```python
from build123d import *

# Parameters (mm, degrees)
SKETCH138_R     = 5
PAD002_DEPTH    = 2
SKETCH139_W     = 64
SKETCH139_H     = 1
SKETCH139_W_2   = 1.03067
SKETCH139_H_2   = 2.2409
SKETCH139_W_3   = 1.02889
SKETCH139_H_3   = 2.288
PAD003_DEPTH    = 65.5
SKETCH140_R     = 5
PAD004_DEPTH    = 2
SKETCH141_W     = 64
SKETCH141_H     = 1
PAD005_DEPTH    = 30
SKETCH144_W     = 28
SKETCH144_H     = 2
PAD007_DEPTH    = 15
SKETCH146_W     = 18.3
SKETCH146_H     = 4.3
POCKET028_DEPTH = 2
FILLET005_R     = 4
FILLET006_R     = 6
SKETCH147_R     = 0.65
POCKET029_DEPTH = 2
SKETCH149_W     = 3.03
SKETCH149_H     = 2.00511
SKETCH149_W_2   = 6
SKETCH149_H_2   = 3
SKETCH149_W_3   = 3.03002
SKETCH149_H_3   = 2.04501
PAD008_DEPTH    = 13.5
SKETCH150_W     = 90
SKETCH150_H     = 24
PAD009_DEPTH    = 2
FILLET007_R     = 9
FILLET008_R     = 5
SKETCH161_W     = 26
SKETCH161_H     = 18
PAD014_DEPTH    = 9
SKETCH162_W     = 23
SKETCH162_H     = 14.90769
SKETCH162_W_2   = 22.99998
SKETCH162_H_2   = 14.95065
POCKET035_DEPTH = 9.5
FILLET014_R     = 2
FILLET015_R     = 2
FILLET016_R     = 1
SKETCH163_R     = 0.75
POCKET036_DEPTH = 2


with BuildPart() as part:
    # Sketch138 → Pad002 (new body)
    with BuildSketch(Plane.XZ):
        with BuildLine():
            ThreePointArc((413.000007, 21.499985), (403.500007, 11.999985), (413.000007, 2.499985))
            Line((477.000007, 2.499985), (413.000007, 2.499985))
            ThreePointArc((477.000007, 2.499985), (486.500006, 11.999985), (477.000007, 21.499985))
            Line((413.000007, 21.499985), (477.000007, 21.499985))
        make_face()
        with Locations((414.971964, 12)):
            Circle(SKETCH138_R, mode=Mode.SUBTRACT)
        with Locations((434.971964, 12)):
            Circle(SKETCH138_R, mode=Mode.SUBTRACT)
        with Locations((454.971964, 12)):
            Circle(SKETCH138_R, mode=Mode.SUBTRACT)
        with Locations((474.982974, 12)):
            Circle(SKETCH138_R, mode=Mode.SUBTRACT)
    extrude(amount=PAD002_DEPTH)

    # Sketch139 (on Face10 of Pad002) → Pad003 (join)
    with BuildSketch(Plane.XZ.offset(2)):
        with Locations((445.000007, 3)):
            Rectangle(SKETCH139_W, SKETCH139_H)
        with Locations((404.084671, 12.02045)):
            Rectangle(SKETCH139_W_2, SKETCH139_H_2)
        with Locations((485.914449, 11.999413)):
            Rectangle(SKETCH139_W_3, SKETCH139_H_3)
    extrude(amount=PAD003_DEPTH)

    # Sketch140 (on Face24 of Pad003) → Pad004 (join)
    with BuildSketch(Plane.XZ.offset(67.5)):
        with BuildLine():
            ThreePointArc((413.000007, 21.499985), (403.500007, 11.999985), (413.000007, 2.499985))
            Line((477.000007, 2.499985), (413.000007, 2.499985))
            ThreePointArc((477.000007, 2.499985), (486.500006, 11.999985), (477.000007, 21.499985))
            Line((413.000007, 21.499985), (477.000007, 21.499985))
        make_face()
        with Locations((414.971964, 12)):
            Circle(SKETCH140_R, mode=Mode.SUBTRACT)
        with Locations((434.971964, 12)):
            Circle(SKETCH140_R, mode=Mode.SUBTRACT)
        with Locations((454.971964, 12)):
            Circle(SKETCH140_R, mode=Mode.SUBTRACT)
        with Locations((474.982974, 12)):
            Circle(SKETCH140_R, mode=Mode.SUBTRACT)
    extrude(amount=PAD004_DEPTH)

    # Sketch141 (on Face32 of Pad004) → Pad005 (join)
    with BuildSketch(Plane(origin=(0, 0, 0), x_dir=(1, 0, 0), z_dir=(0, 1, 0))):
        with Locations((445, -3.005366)):
            Rectangle(SKETCH141_W, SKETCH141_H)
    extrude(amount=PAD005_DEPTH)

    # Sketch144 (on Face35 of Pad005) → Pad007 (join)
    with BuildSketch(Plane(origin=(0, 0, 3.505366), x_dir=(-1, 0, 0), z_dir=(0, 0, 1))):
        with Locations((-445, -28)):
            Rectangle(SKETCH144_W, SKETCH144_H)
    extrude(amount=PAD007_DEPTH)

    # Sketch146 (on Face41 of Pad007) → Pocket028 (cut)
    with BuildSketch(Plane(origin=(0, 29, 0), x_dir=(1, 0, 0), z_dir=(0, 1, 0))):
        with Locations((444.99999, -12)):
            Rectangle(SKETCH146_W, SKETCH146_H)
    extrude(amount=-POCKET028_DEPTH, mode=Mode.SUBTRACT)

    # Fillet005
    fillet005_edges = [part.edges().sort_by_distance(p)[0] for p in [
        (431, 28, 18.505366),
        (459, 28, 18.505366),
    ]]
    fillet(fillet005_edges, radius=FILLET005_R)

    # Fillet006
    fillet006_edges = [part.edges().sort_by_distance(p)[0] for p in [
        (431, 28, 3.505366),
        (459, 28, 3.505366),
    ]]
    fillet(fillet006_edges, radius=FILLET006_R)

    # Sketch147 (on Face5 of Fillet006) → Pocket029 (cut)
    with BuildSketch(Plane(origin=(0, 29, 0), x_dir=(1, 0, 0), z_dir=(0, 1, 0))):
        with Locations((434.559988, -12)):
            Circle(SKETCH147_R)
        with Locations((455.43999, -12)):
            Circle(SKETCH147_R)
    extrude(amount=-POCKET029_DEPTH, mode=Mode.SUBTRACT)

    # Sketch149 (on Face52 of Pocket029) → Pad008 (join)
    with BuildSketch(Plane.XZ.offset(69.5)):
        with Locations((484.914989, 12.142557)):
            Rectangle(SKETCH149_W, SKETCH149_H)
        with Locations((445, 4.5)):
            Rectangle(SKETCH149_W_2, SKETCH149_H_2)
        with Locations((405.084996, 12.122505)):
            Rectangle(SKETCH149_W_3, SKETCH149_H_3)
        with Locations((445.000007, 19.5)):
            Rectangle(SKETCH149_W_2, SKETCH149_H_2)
    extrude(amount=PAD008_DEPTH)

    # Sketch150 (on Face70 of Pad008) → Pad009 (join)
    with BuildSketch(Plane.XZ.offset(83)):
        with Locations((444.999989, 12.25)):
            Rectangle(SKETCH150_W, SKETCH150_H)
    extrude(amount=PAD009_DEPTH)

    # Fillet007
    fillet007_edges = [part.edges().sort_by_distance(p)[0] for p in [
        (489.999989, -84, 24.25),
        (399.999989, -84, 24.25),
    ]]
    fillet(fillet007_edges, radius=FILLET007_R)

    # Fillet008
    fillet008_edges = [part.edges().sort_by_distance(p)[0] for p in [
        (489.999989, -84, 0.25),
        (399.999989, -84, 0.25),
    ]]
    fillet(fillet008_edges, radius=FILLET008_R)

    # Sketch161 (on Face1 of Fillet008) → Pad014 (join)
    with BuildSketch(Plane(origin=(0, -83, 0), x_dir=(1, 0, 0), z_dir=(0, 1, 0))):
        with Locations((467, -12.257592)):
            Rectangle(SKETCH161_W, SKETCH161_H)
        with Locations((422.99999, -12.250199)):
            Rectangle(SKETCH161_W, SKETCH161_H)
    extrude(amount=PAD014_DEPTH)

    # Sketch162 (on Face34 of Pad014) → Pocket035 (cut)
    with BuildSketch(Plane.XZ.offset(85)):
        with Locations((423.000006, 12.246182)):
            Rectangle(SKETCH162_W, SKETCH162_H)
        with Locations((466.999997, 12.225325)):
            Rectangle(SKETCH162_W_2, SKETCH162_H_2)
    extrude(amount=-POCKET035_DEPTH, mode=Mode.SUBTRACT)

    # Fillet014
    fillet014_edges = [part.edges().sort_by_distance(p)[0] for p in [
        (434.500006, -75.5, 12.246182),
        (455.500007, -75.5, 12.225325),
    ]]
    fillet(fillet014_edges, radius=FILLET014_R)

    # Fillet015
    fillet015_edges = [part.edges().sort_by_distance(p)[0] for p in [
        (455.500007, -81.25, 4.75),
        (434.500006, -81.25, 4.792337),
        (434.500006, -81.25, 19.700027),
        (455.500007, -81.25, 19.70065),
    ]]
    fillet(fillet015_edges, radius=FILLET015_R)

    # Fillet016
    fillet016_edges = [part.edges().sort_by_distance(p)[0] for p in [
        (411.500006, -81.25, 4.792337),
        (411.500006, -75.5, 12.246182),
        (411.500006, -81.25, 19.700027),
        (411.500006, -76.085786, 19.114241),
        (411.500006, -76.085786, 5.378123),
        (478.499987, -81.25, 4.75),
        (478.499987, -76.085786, 5.335786),
        (478.499987, -75.5, 12.225325),
        (478.499987, -76.085786, 19.114864),
        (478.499987, -81.25, 19.70065),
    ]]
    fillet(fillet016_edges, radius=FILLET016_R)

    # Sketch163 (on Face2 of Fillet016) → Pocket036 (cut)
    with BuildSketch(Plane.XZ.offset(85)):
        with Locations((403.000006, 19.8)):
            Circle(SKETCH163_R)
        with Locations((487.03999, 19.8)):
            Circle(SKETCH163_R)
        with Locations((402.069775, 3.2)):
            Circle(SKETCH163_R)
        with Locations((488.100007, 3.2)):
            Circle(SKETCH163_R)
    extrude(amount=-POCKET036_DEPTH, mode=Mode.SUBTRACT)


with BuildPart() as part_1:
    # Body015 placement: moved
    add(part.part.moved(Location((0, 182, 0))))


solid = part_1.part
```
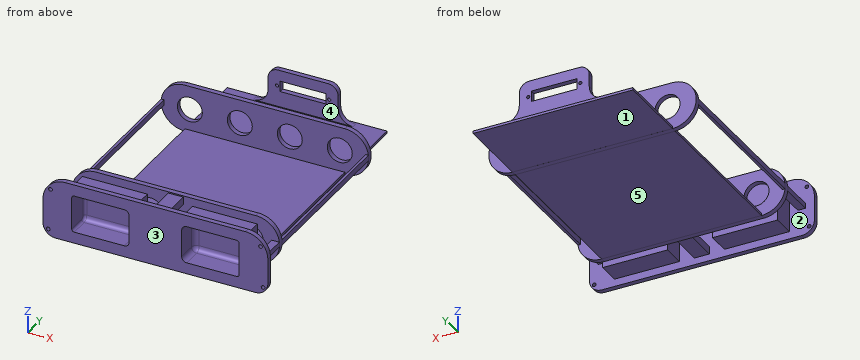
Check sheet for the modelled part. Datum: model origin and axes. Units: mm. Face numbers are marked on the shaded views. A direction names the side the tool comes from. Coordinates: 2 decimals unless noted, no trailing zeros. Loops run counter-clockwise (first coordinate to the right, second up) from the corner with the lowest first, then second, coordinate; pieces in that order, holes last.
1) Material ranges on probe 1 along X at (y, z) = (210.6, 12); probe 2 along Y at (x, z) = (405, 12.5); probe 3 along Y at (x, z) = (409, 10.5), recorded low to high.
2) Gauge pin test, flat ends, axial feed: pin 1 (5 mm diameter, centred on y = 131, z = 10, fed in from +X); pin 2 (1.5 mm diameter, centred on y = 111.5, z = 7.5, fed in from +X); pin 3 (7 mm diameter, centred on y = 103, z = 11.5, fed in from -X); pin 4 (13 mm diameter, centred on x = 474.98, z = 12, fed in from +Y). Record the tip position at first contact, or that the pin passes through.
3) Release check for a two-part mould opening along X. For the marked faces 1 and 2 record: released by +X, released by -X, zero draft, split by the parting line, or undercut.
4) Access from +Z, -Z, +X, -X, +Y, -Y to the whole of each face (thin tool, end or side, straight path). Record for the marked faces 3, 4 and 5.
5) Sectioned sample at A-A (y = 146.5). Record the boundary of the cut face in (x, z).
Check sheet entries:
1. probe 1: x = 431 to 433.91, 435.21 to 435.85, 454.15 to 454.79, 456.09 to 459
1. probe 2: y = 97 to 114.5, 180 to 182
1. probe 3: y = 97 to 99, 112.5 to 114.5, 180 to 182
2. pin 1: stops at x = 486.43
2. pin 2: passes through
2. pin 3: stops at x = 403.57
2. pin 4: stops at y = 182
3. face 1: zero draft
3. face 2: undercut
4. face 3: +Z, -Z, +X, -X, -Y
4. face 4: +Z, +X, -X
4. face 5: -Z, +X, -X, +Y
5. outline: (403.57, 10.9) - (404.6, 10.9) - (404.6, 13.14) - (403.57, 13.14) - close; (413, 2.5) - (477, 2.5) - (477, 3.5) - (413, 3.5) - close; (485.4, 10.86) - (486.43, 10.86) - (486.43, 13.14) - (485.4, 13.14) - close
